Part model, mm, in its own coordinate system. A direction names the side the tool comes from. Round coordinates to 2 decimals unless told otherwise and drop trailing zeros. Write each loop counter-clockwise with the first axis right and the second up, starting at its lowest first coordinate (ties: lowest second). Pieces come first, ordered by that corner, then holes.
```python
from build123d import *
from build123d.topology import SkipClean

# Parameters (mm, degrees)
SKETCH2_R           = 3.175
BOSS_EXTRUDE1_DEPTH = 12.7
SKETCH3_R           = 4.445
BOSS_EXTRUDE2_DEPTH = 2.032
THREAD1_PITCH       = 1.27


with BuildPart() as part:
    # Sketch2 → Boss-Extrude1 (new body)
    with BuildSketch(Plane(origin=(0, 0, 0), x_dir=(1, 0, 0), z_dir=(0, 1, 0))):
        with Locations(Location((0, 0, 0), (0, 0, 270))):
            Circle(SKETCH2_R)
    extrude(amount=BOSS_EXTRUDE1_DEPTH)

    # Sketch3 → Boss-Extrude2 (add)
    with BuildSketch(Plane(origin=(0, 0, 0), x_dir=(-1, 0, 0), z_dir=(0, -1, 0))):
        with Locations(Location((0, 0, 0), (0, 0, 90))):
            Circle(SKETCH3_R)
    extrude(amount=BOSS_EXTRUDE2_DEPTH)

    # Thread1: the profile of Thread Profile1 profile screwed along a right-hand helix of 3.75 turns, 8 arcs to a turn; built about Z, then put on its axis
    with SkipClean():  # the faces are left unmerged after this step: merging them gives an invalid solid
        thread1_z = Axis((0, 0, 0), (0, 0, 1))
        thread1_corners = [(3.1747, 0, -0.000173205), (3.1747, 0, 1.111423202), (3.862407661, 0, 0.714374998), (3.862407661, 0, 0.396874998)]
        with BuildLine(mode=Mode.PRIVATE) as thread1_profile:
            Line(thread1_corners[0], thread1_corners[1])
            Line(thread1_corners[1], thread1_corners[2])
            Line(thread1_corners[2], thread1_corners[3])
            Line(thread1_corners[3], thread1_corners[0])
        thread1_cap = Face(thread1_profile.wire())
        thread1_turn_angles = [0, 22.5, 45, 67.5, 90, 112.5, 135, 157.5, 180, 202.5, 225, 247.5, 270, 292.5, 315, 337.5, 360]
        thread1_turn_weights = [1, 0.9238795325112867, 1, 0.9238795325112867, 1, 0.9238795325112867, 1, 0.9238795325112867, 1, 0.9238795325112867, 1, 0.9238795325112867, 1, 0.9238795325112867, 1, 0.9238795325112867, 1]
        thread1_turn_rails = [Edge.make_bspline([Vector(p[0], p[1], 0).rotate(thread1_z, thread1_turn_angles[k]) / thread1_turn_weights[k] + Vector(0, 0, p[2] + THREAD1_PITCH * thread1_turn_angles[k] / 360) for k in range(17)], [0, 0, 0, 1, 1, 2, 2, 3, 3, 4, 4, 5, 5, 6, 6, 7, 7, 8, 8, 8], 2, thread1_turn_weights) for p in thread1_corners]
        thread1_turn_sides = [Face.make_surface_from_curves(thread1_turn_rails[p[0]], thread1_turn_rails[p[1]]) for p in [(0, 1), (1, 2), (2, 3), (3, 0)]]
        thread1_last_angles = [1080, 1102.5, 1125, 1147.5, 1170, 1192.5, 1215, 1237.5, 1260, 1282.5, 1305, 1327.5, 1350]
        thread1_last_weights = [1, 0.9238795325112867, 1, 0.9238795325112867, 1, 0.9238795325112867, 1, 0.9238795325112867, 1, 0.9238795325112867, 1, 0.9238795325112867, 1]
        thread1_last_rails = [Edge.make_bspline([Vector(p[0], p[1], 0).rotate(thread1_z, thread1_last_angles[k]) / thread1_last_weights[k] + Vector(0, 0, p[2] + THREAD1_PITCH * thread1_last_angles[k] / 360) for k in range(13)], [0, 0, 0, 1, 1, 2, 2, 3, 3, 4, 4, 5, 5, 6, 6, 6], 2, thread1_last_weights) for p in thread1_corners]
        thread1_last_sides = [Face.make_surface_from_curves(thread1_last_rails[p[0]], thread1_last_rails[p[1]]) for p in [(0, 1), (1, 2), (2, 3), (3, 0)]]
        thread1 = Plane(origin=(0, 0, 0), x_dir=(1, 0, 0), z_dir=(0, 1, 0)) * Solid(Shell([*[p.moved(Location((0, 0, THREAD1_PITCH * i))) for i in range(3) for p in thread1_turn_sides], *thread1_last_sides, thread1_cap, thread1_cap.rotate(thread1_z, 1350).moved(Location((0, 0, THREAD1_PITCH * 1350 / 360)))]))
        add(thread1)


solid = part.part
```
Q1. Which spindle directions (+Z, -Z, +X, -X, +Y, -Y) get a long thin tool onto all of the face, cutting with end or side? Do faces 1 (the cylindrical face through (-4.34, -1, 0.96)), 2 (the flat face through (-3, 0, -2)). Say none if no direction does.
Values follow:
face 1: +Y, -Y
face 2: none
Q2. Cut at B-B on z = 3.5. State how many separate pieces and enclosed holes the cut face has, plus the area to 3 significant figures.
Values follow:
separate pieces: 5
enclosed holes: 0
area: 17.9 mm2
Q3. Cut at A-A on y = 8. Write the cut outline in (x, z) (3 decimals).
Values follow:
outline: circle Ø6.35 at (0, 0)
Q4. Drop flat-ended pins along their axis: pin 1 (5 mm diameter, centred on y = 3, z = 0, fed in from -X); pin 2 (4 mm diameter, centred on x = 1, y = 9.5, fed in from +Z) (3 decimals); pin 3 (5 mm diameter, centred on x = -3, y = 2, fed in from +Z). Give the stop position or say it passes through.
Values follow:
pin 1: stops at x = -3.86
pin 2: stops at z = 3.175
pin 3: stops at z = 4.18
Q5. Wall check: L1, parallel to Y at x = -1, z = -3.5; L2, parallel to Y at x = -1, z = 3.5; L3, parallel to Y at x = -2.25, z = 3.5. Give the ranges that are in metal, low to high.
Values follow:
L1: y = -2.03 to 0, 0.64 to 1.22, 1.91 to 2.49, 3.18 to 3.76, 4.45 to 5.03
L2: y = -2.03 to 0, 1.17 to 1.74, 2.44 to 3.01, 3.71 to 4.28, 4.98 to 5.55
L3: y = -2.03 to 0
Q6. Cut at C-C on y = -1. Write the cut outline in (x, z) (3 decimals), plus the area to 3 significant figures.
Values follow:
outline: circle Ø8.89 at (0, 0)
area: 62.1 mm2
